from build123d import *

# Parameters (mm, degrees)
BOSS_EXTRUDE1_DEPTH = 615
SKETCH2_R           = 4
CUT_EXTRUDE1_DEPTH  = 5


with BuildPart() as part:
    # Sketch1 → Boss-Extrude1 (new body)
    with BuildSketch(Plane.XY):
        with BuildLine():
            Line((-12.5, 5), (12.5, 5))
            ThreePointArc((12.5, 5), (17.5, 0), (12.5, -5))
            Line((12.5, -5), (-12.5, -5))
            ThreePointArc((-12.5, -5), (-17.5, 0), (-12.5, 5))
        make_face()
    extrude(amount=-BOSS_EXTRUDE1_DEPTH)

    # Sketch2 → Cut-Extrude1 (cut)
    with BuildSketch(Plane.XZ.offset(5)):
        with Locations(Location((0, -15, 0), (0, 0, 270))):
            Circle(SKETCH2_R)
        with Locations(Location((0, -600, 0), (0, 0, 270))):
            Circle(SKETCH2_R)
    extrude(amount=-CUT_EXTRUDE1_DEPTH, mode=Mode.SUBTRACT)


solid = part.part
Part model, mm, in its own coordinate system. Give positions to 0.01 mm unless a question says otherwise; leave off trailing zeros. Order: outer loops, then holes, each group sorted by start corner. A loop starts at its lowest first (then second) coordinate and runs counter-clockwise, first axis right, second up. Notation, with made-up numbers: (-37, -18.75) - (5, -18.75) arc R32 ccw to (5, 7.25) - close; hole circle Ø3 at (49.25, -20.75). An arc over 180 degrees is marked (long way). Use a Markdown table: item, result.
1) Saw through at B-B on y = 3.5. List the corners of the cut face in (x, z), plus the area to 3 significant figures.
Checked values:
| item | result |
|---|---|
| outline | (-16.07, -615) - (16.07, -615) - (16.07, 0) - (-16.07, 0) - close |
| area | 19,800 mm² |
2) Flat gauge pin, fed straight in: P1, Ø7, axis at x = 0, z = -15, coming from the -Y side. Where does the tip first touch, or does it go through?
Checked values:
| item | result |
|---|---|
| P1 | y = 0 |
3) Probe L1, parallel to X at y = -0.75, z = -523; L2, parallel to Z at x = 2.5, y = -2.5; L3, parallel to X at y = 0.5, z = -446.5. List the from-to ranges inside material, lowest first. Write a range as from..to.
Checked values:
| item | result |
|---|---|
| L1 | -17.44..17.44 |
| L2 | -615..-603.12, -596.88..-18.12, -11.88..0 |
| L3 | -17.47..17.47 |
4) Saw through at A-A on z = -207.5. List the corners of the cut face in (x, y).
Checked values:
| item | result |
|---|---|
| outline | (-12.5, -5) - (12.5, -5) arc R5 ccw to (12.5, 5) - (-12.5, 5) arc R5 ccw to start |
